Here's the drawing with two shaded views (mm, measured from the low corner). I have some questions. A direction names the side the tool comes from. Round coordinates to 2 decimals unless told otherwise and drop trailing zeros. Loops run counter-clockwise (first coordinate to the right, second up) from the corner with the lowest first, then second, coordinate; pieces in that order, holes last. Notation, with made-up numbers: M 3,11.5 L 27,11.5 A23 cw 27,21.5 Z; hole C 69.5,84 d11. An arc over 180 degrees is marked long. Answer as a JSON object with one key per item and string values.
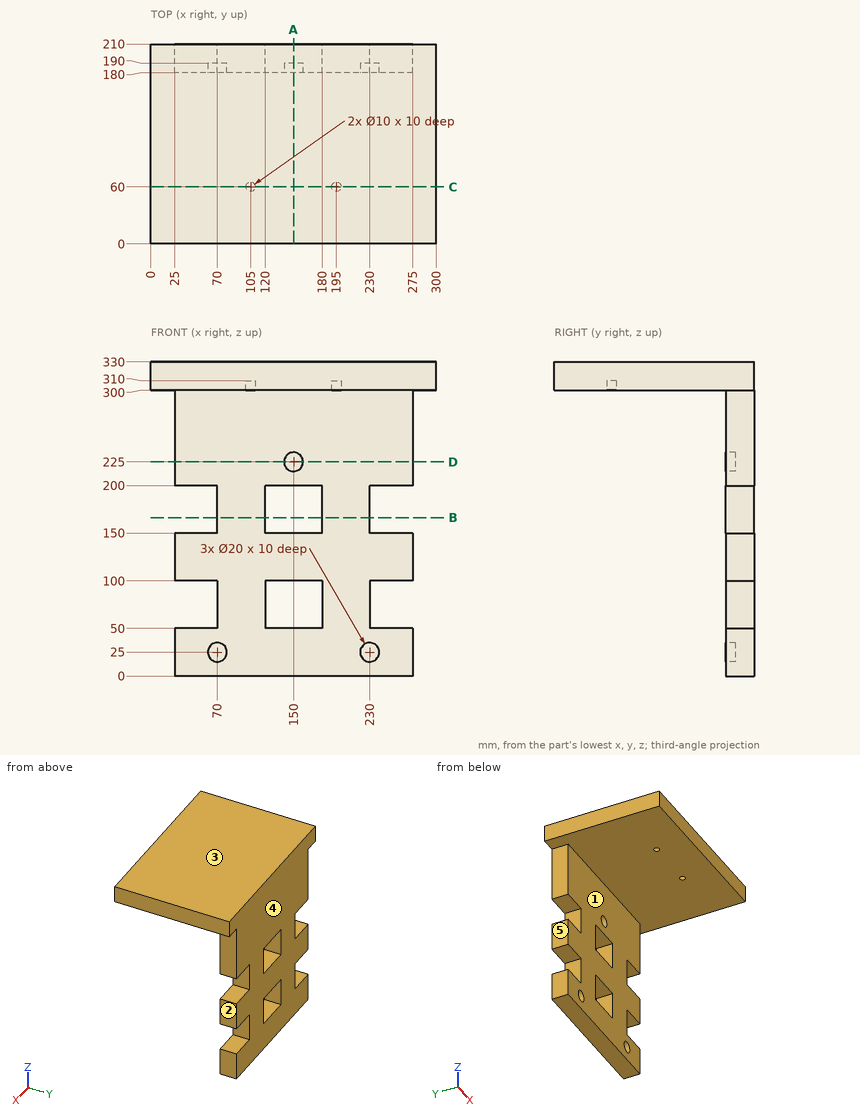
Item 1: I want a section at B-B on z = 166.5. List the corners of the cut face in (x, y) for me, plus the area to 3 significant figures.
Solution:
{"outline": "M 70,180 L 120,180 L 120,210 L 70,210 Z; M 180,180 L 230,180 L 230,210 L 180,210 Z", "area": "3,000 mm2"}
Item 2: For P1, Ø9, axis at x = 105, y = 60, coming from the -Z side; P2, Ø9, axis at y = 190, z = 238, coming from the +X side; P3, Ø6, axis at x = 213.5, z = 191.5, coming from the -Y side, each with a flat end and sliding along its axis, tell me the tip position at first contact or that it passes through.
Solution:
{"P1": "stops at z = 310", "P2": "stops at x = 275", "P3": "stops at y = 180"}
Item 3: I want a section at D-D on z = 225. List the corners of the cut face in (x, y) for me, plus the area to 3 significant figures.
Solution:
{"outline": "M 25,180 L 140,180 L 140,190 L 160,190 L 160,180 L 275,180 L 275,210 L 25,210 Z", "area": "7,300 mm2"}
Item 4: For the marked faces 1, 2, 3, 4 and 5, which set-ups out of +Z, -Z, +X, -X, +Y, -Y let a thin tool reach every point of the face, with its end or its side?
Solution:
{"face 1": "-Z, +X, -X, -Y", "face 2": "-Z, +X, +Y, -Y", "face 3": "+Z, +X, -X, +Y, -Y", "face 4": "+Z, -Z, +X, -X, +Y", "face 5": "-Z, -X, +Y, -Y"}
Item 5: If I drill on L1, parallel to Y at x = 105, z = 302.5; L2, parallel to X at y = 199, z = 151.5; L3, parallel to Z at x = 242, y = 57.5, over which ranges is the centre line in solid material (lowest first)? Write a range as from..to.
Solution:
{"L1": "y = 0..55, 65..210", "L2": "x = 70..120, 180..230", "L3": "z = 300..330"}
Item 6: I want a section at A-A on x = 150. List the corners of the cut face in (y, z) for me.
Solution:
{"outline": "M 0,300 L 180,300 L 180,235 L 190,235 L 190,215 L 180,215 L 180,200 L 210,200 L 210,330 L 0,330 Z; M 180,0 L 210,0 L 210,50 L 180,50 Z; M 180,100 L 210,100 L 210,150 L 180,150 Z"}
Item 7: I want a section at C-C on y = 60. List the corners of the cut face in (x, z) for me, plus the area to 3 significant figures.
Solution:
{"outline": "M 0,300 L 100,300 L 100,310 L 110,310 L 110,300 L 190,300 L 190,310 L 200,310 L 200,300 L 300,300 L 300,330 L 0,330 Z", "area": "8,800 mm2"}
